Could you check a few things on this model? Use its own coordinates, in mm. A direction names the side the tool comes from. Round coordinates to 2 decimals unless told otherwise and drop trailing zeros. Loops run counter-clockwise (first coordinate to the right, second up) from the corner with the lowest first, then second, coordinate; pieces in that order, holes last. Notation, with made-up numbers: (83, 29.25) -> (133, 29.25) arc R23 cw to (133, 56.25) -> close; hole circle Ø2 at (-3.75, 73). An arc over 180 degrees is marked (long way). One line per item, written item: value.
Autodesk Inventor part; units mm, degrees
ref_plane "YZ Plane" through (0, 0, 0) normal (1, 0, 0) x (0, 1, 0)
ref_plane "XZ Plane" through (0, 0, 0) normal (0, 1, 0) x (-1, 0, 0)
ref_plane "XY Plane" through (0, 0, 0) normal (0, 0, 1) x (1, 0, 0)
sketch "Sketch1" plane through (0, 0, 0) normal (0, 1, 0) x (-1, 0, 0)
  line L0 (-19, -19) -> (19, -19)
  line L1 (19, -19) -> (19, 19)
  line L2 (19, 19) -> (-19, 19)
  line L3 (-19, 19) -> (-19, -19)
  line L4 (-19, -19) -> (19, 19) construction
  line L5 (19, -19) -> (-19, 19) construction
  point P0 (0, 0)
  dimension "d0" = 38
  dimension "d1" = 38
extrude "Extrusion1" add sketch "Sketch1" along normal blind 5
sketch "Sketch5" plane through (0, 5, 0) normal (0, 1, 0) x (1, 0, 0)
  line L0 (-19, -19) -> (19, -19)
  line L1 (-19, 19) -> (19, 19)
  line L2 (19, 19) -> (19, -19)
  line L3 (19, -19) -> (-19, -19)
  line L4 (-19, -19) -> (-19, 19)
  line L5 (-19, 19) -> (19, -19) construction
  line L6 (19, 19) -> (-19, -19) construction
  point P0 (0, 0)
extrude "Extrusion5" add sketch "Sketch5" along normal blind 800
sketch "Sketch6" plane through (0, 805, 0) normal (0, 1, 0) x (1, 0, 0)
  line L0 (-7.5, 27.5) -> (7.5, 27.5)
  line L1 (7.5, -27.5) -> (-7.5, -27.5)
  line L2 (-7.5, 27.5) -> (7.5, -27.5) construction
  line L3 (7.5, 27.5) -> (-7.5, -27.5) construction
  line L4 (-27.5, 7.5) -> (-27.5, -7.5)
  line L5 (27.5, -7.5) -> (27.5, 7.5)
  line L6 (27.5, 7.5) -> (-27.5, -7.5) construction
  line L7 (-27.5, 7.5) -> (27.5, -7.5) construction
  line L8 (-27.5, -7.5) -> (-7.5, -7.5)
  line L9 (7.5, -7.5) -> (27.5, -7.5)
  line L10 (7.5, 27.5) -> (7.5, 7.5)
  line L11 (7.5, -7.5) -> (7.5, -27.5)
  line L12 (27.5, 7.5) -> (7.5, 7.5)
  line L13 (-7.5, 7.5) -> (-27.5, 7.5)
  line L14 (-7.5, -27.5) -> (-7.5, -7.5)
  line L15 (-7.5, 7.5) -> (-7.5, 27.5)
  point P0 (0, 0)
  dimension "d20" = 15
  dimension "d21" = 55
  dimension "d22" = 55
  dimension "d23" = 15
sketch "Sketch7" plane through (0, 805, 0) normal (0, 1, 0) x (1, 0, 0)
  line L0 (-17.5, 17.5) -> (17.5, 17.5)
  line L1 (17.5, 17.5) -> (17.5, -17.5)
  line L2 (17.5, -17.5) -> (-17.5, -17.5)
  line L3 (-17.5, -17.5) -> (-17.5, 17.5)
  line L4 (-17.5, 17.5) -> (17.5, -17.5) construction
  line L5 (17.5, 17.5) -> (-17.5, -17.5) construction
  point P0 (0, 0)
  dimension "d24" = 35
  dimension "d25" = 35
extrude "Extrusion6" cut sketch "Sketch7" against normal blind 800
extrude "Extrusion7" cut sketch "Sketch6" against normal blind 800
sketch "Sketch8" plane through (0, 5, 0) normal (0, 1, 0) x (1, 0, 0)
  circle A0 centre (0, 0) radius 5
  dimension "d30" = 10
extrude "Extrusion8" cut sketch "Sketch8" against normal blind 2
sketch "Sketch9" plane through (-19, 0, 19) normal (0, 0, 1) x (1, 0, 0)
  line L0 (-0.2068, 780.9612) -> (38, 780.9612) construction
  line L1 (38, 0) -> (38, 805)
  circle A0 centre (18.8966, 780.9612) radius 6.5
  circle A1 centre (18.8966, 780.9612) radius 12.454
  point P0 (19, 0)
  dimension "d33" = 13
extrude "Extrusion9" add sketch "Sketch9" along normal blind 20
properties part number "marble_lift_outer"
(1) If I drill on L1, parallel to Z at x = 16, y = 179.5; L2, parallel to Y at x = -13.5, z = -13.5, over which ranges is the centre line in solid material (lowest first)?
Recorded:
L1: -19 to -17.5, 17.5 to 19
L2: 0 to 5
(2) If we section it at A-A, the plane y = 219: Please give me the cut outline in (x, z), then the cut area to 3 significant figures.
Recorded:
outline: (-19, -19) -> (-7.5, -19) -> (-7.5, -17.5) -> (-17.5, -17.5) -> (-17.5, -7.5) -> (-19, -7.5) -> close; (-19, 7.5) -> (-17.5, 7.5) -> (-17.5, 17.5) -> (-7.5, 17.5) -> (-7.5, 19) -> (-19, 19) -> close; (7.5, -19) -> (19, -19) -> (19, -7.5) -> (17.5, -7.5) -> (17.5, -17.5) -> (7.5, -17.5) -> close; (7.5, 17.5) -> (17.5, 17.5) -> (17.5, 7.5) -> (19, 7.5) -> (19, 19) -> (7.5, 19) -> close
area: 129 mm²
(3) For faces 1 (the face through (-1.725, 768.613, 28.86)), 2 (the face through (-3, 787, 19)), 3 (the face through (5, 776, 39)), which set-ups out of +Z, -Z, +X, -X, +Y, -Y let a thin tool reach every point of the face, with its end or its side?
Recorded:
face 1: +Z
face 2: -Z, +Y
face 3: +Z, +X, -X, +Y, -Y
(4) Thinking about a two-plate mould opening in Y: for faces 4 (the face through (-8, 397, -19)), 5 (the face through (0, 0, 0)), 6 (the face through (-0.95, 774.517, 28.86)), which applies, released by +Y, released by -Y, zero draft, split by the parting line, or undercut?
Recorded:
face 4: zero draft
face 5: released by -Y
face 6: undercut
(5) If we section it at B-B, the plane z = 27: Please give me the cut outline in (x, y).
Recorded:
outline: circle Ø24.91 at (-0.1, 780.96); hole circle Ø13 at (-0.1, 780.96)
(6) I'm going to push flat-ended pins straight in: pin 1 Ø10 at (x, z) = (9.5, 31) entering from +Y; pin 2 Ø11.5 at (x, y) = (2, 427.5) entering from +Z; pin 3 Ø8 at (x, z) = (-1.5, 0) entering from +Y. Where does each tip first touch, or does it pass through?
Recorded:
pin 1: y = 792.53
pin 2: z = 19
pin 3: y = 5
